Can you work these out from the drawing? Everything is in mm from the part's minimum corner. A direction names the side the tool comes from. Give positions to 0.01 mm unless a question says otherwise; leave off trailing zeros. Loops run counter-clockwise (first coordinate to the right, second up) from the corner with the lowest first, then second, coordinate; pieces in that order, holes last. Notation, with made-up numbers: (80.25, 1.5) - (113.25, 1.5) arc R30 cw to (113.25, 26.5) - close; hole circle Ø9 at (57, -31). An arc over 180 degrees is marked (long way). Write each question's results on one line, items separated by ' | '. Start each with the question number.
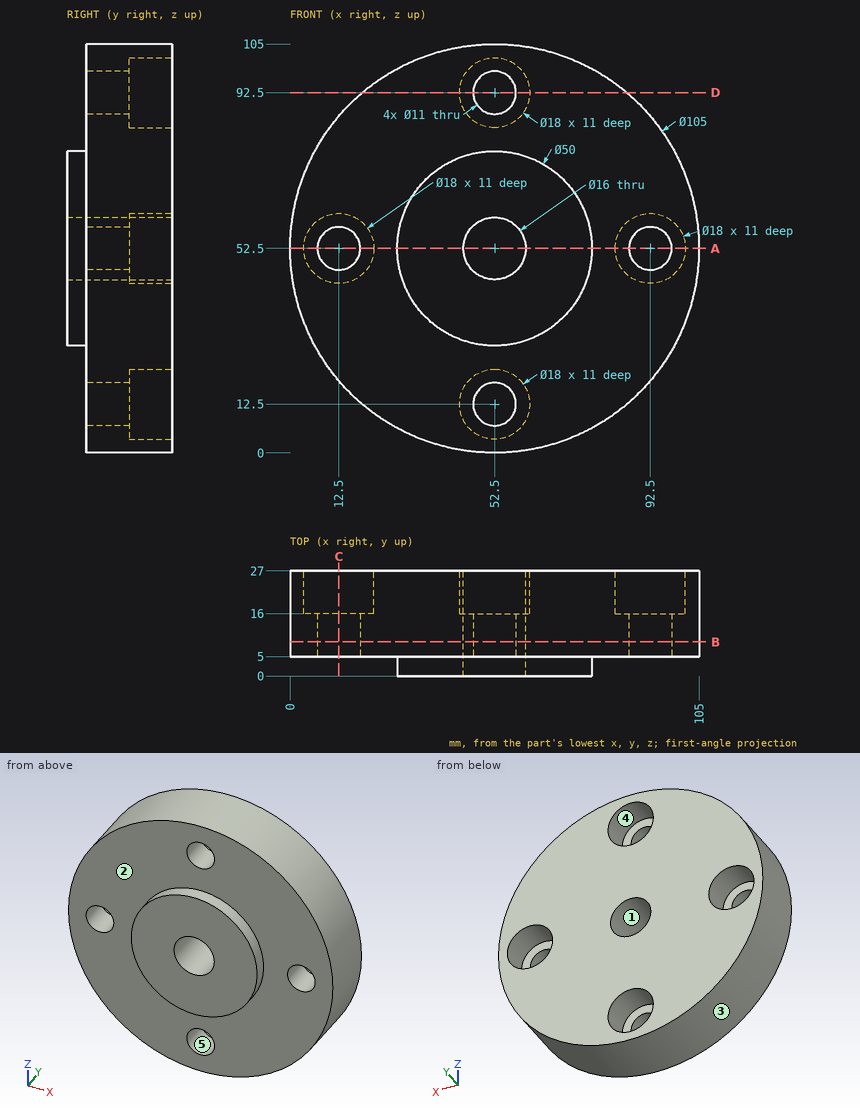
Q1. I need wall thicknesses on L1, parallel to X at y = 10.5, z = 54; L2, parallel to X at y = 23.5, z = 58.5; L3, parallel to X at y = 7.5, z = 12.5. Which ranges of each line are inside material? Lowest first, please. Write a range as from..to.
Q2. I want a section at D-D, the plane z = 92.5. List the corners of the cut face in (x, y) for me.
Q3. I want a section at C-C, the plane x = 12.5. List the corners of the cut face in (y, z) for me, then the cut area to 3 significant figures.
Q4. I'm going to push flat-ended pins straight in: pin 1 Ø12 at (x, z) = (31.5, 64) entering from -Y; pin 2 Ø16 at (x, z) = (52.5, 92.5) entering from -Y; pin 3 Ø9 at (x, z) = (52.5, 12.5) entering from +Y; pin 4 Ø16 at (x, z) = (92.5, 52.5) entering from +Y. Where does each tip first touch, or does it pass through?
Q5. Which directions (+Z, -Z, +X, -X, +Y, -Y) give clear straight access to the entire face, cutting with the end or side of a thin tool? Please do the marked faces 4 and 5.
Q6. I want a section at B-B, the plane y = 8.75. List the corners of the cut face in (x, z) for me, then the cut area to 3 significant figures.
Q7. I want a section at A-A, the plane z = 52.5. List the corners of the cut face in (x, y) for me.
Q8. If we mould it in two halves opening along X, with no side actions, what happens to the marked faces 1, 2 and 3? For each: +X half, -X half, draft (parallel to the pull), parting line (faces both ways), or undercut.
Conclusion:
1) L1: 0.02..7.21, 17.79..44.64, 60.36..87.21, 97.79..104.98 | L2: 0.34..5.79, 19.21..47.21, 57.79..85.79, 99.21..104.66 | L3: 18.5..47, 58..86.5
2) outline: (18.5, 5) - (47, 5) - (47, 16) - (43.5, 16) - (43.5, 27) - (18.5, 27) - close; (58, 5) - (86.5, 5) - (86.5, 27) - (61.5, 27) - (61.5, 16) - (58, 16) - close
3) outline: (5, 18.5) - (27, 18.5) - (27, 43.5) - (16, 43.5) - (16, 47) - (5, 47) - close; (5, 58) - (16, 58) - (16, 61.5) - (27, 61.5) - (27, 86.5) - (5, 86.5) - close | area: 1,180 mm^2
4) pin 1: y = 0 | pin 2: y = 5 | pin 3: through | pin 4: y = 16
5) face 4: +Y | face 5: +Y, -Y
6) outline: circle Ø105 at (52.5, 52.5); hole circle Ø11 at (12.5, 52.5); hole circle Ø16 at (52.5, 52.5); hole circle Ø11 at (52.5, 12.5); hole circle Ø11 at (52.5, 92.5); hole circle Ø11 at (92.5, 52.5) | area: 8,080 mm^2
7) outline: (0, 5) - (7, 5) - (7, 16) - (3.5, 16) - (3.5, 27) - (0, 27) - close; (18, 5) - (27.5, 5) - (27.5, 0) - (44.5, 0) - (44.5, 27) - (21.5, 27) - (21.5, 16) - (18, 16) - close; (60.5, 0) - (77.5, 0) - (77.5, 5) - (87, 5) - (87, 16) - (83.5, 16) - (83.5, 27) - (60.5, 27) - close; (98, 5) - (105, 5) - (105, 27) - (101.5, 27) - (101.5, 16) - (98, 16) - close
8) face 1: undercut | face 2: draft | face 3: parting line
